from build123d import *

# Parameters (mm, degrees)
SKETCH_1_W               = 105
SKETCH_1_H               = 105
EXTRUDE_1_DEPTH          = 9
SKETCH_2_R               = 5.5
CUT_EXTRUDE_1_DEPTH      = 9
SKETCH_4_W               = 10
SKETCH_4_H               = 10
EXTRUDE_2_DEPTH          = 30
SKETCH_5_R               = 12.5
EXTRUDE_3_DEPTH          = 10
SKETCH_6_W               = 8
SKETCH_6_H               = 8
EXTRUDE_4_DEPTH          = 380
EXTRUDE_5_DEPTH          = 10
PATTERN_LINEAR_1_COUNT   = 5
PATTERN_LINEAR_1_PITCH   = 80
EXTRUDE_6_DEPTH          = 10
SKETCH_9_W               = 105
SKETCH_9_H               = 15
CUT_EXTRUDE_2_DEPTH      = 59
SPLIT_START              = -31.043560763
SPLIT_BODIES_2_OUTLINE_R = 5.5
SPLIT_BODIES_2_DEPTH     = 40.043560763
SKETCH_10_W              = 8
SKETCH_10_H              = 8
EXTRUDE_8_DEPTH          = 9


# Read off the part's stored shape, not the designer's step: 分割2
with BuildPart() as part:
    # 草图1 → 凸台-拉伸1 (new body)
    with BuildSketch(Plane(origin=(0, 0, 0), x_dir=(1, 0, 0), z_dir=(0, 1, 0))):
        with BuildLine():
            Line((-102.5, 102.5), (102.5, 102.5))
            Line((102.5, 102.5), (146.930137945, 8.550357413))
            ThreePointArc((146.930137945, 8.550357413), (148.85, 0), (146.930137945, -8.550357413))
            Line((146.930137945, -8.550357413), (90, -67.5))
            Line((90, -67.5), (52.5, -67.5))
            Line((52.5, -67.5), (-52.5, -67.5))
            Line((-52.5, -67.5), (-90, -67.5))
            Line((-90, -67.5), (-146.930137945, -8.550357413))
            ThreePointArc((-146.930137945, -8.550357413), (-148.85, 0), (-146.930137945, 8.550357413))
            Line((-146.930137945, 8.550357413), (-102.5, 102.5))
        make_face()
        Rectangle(SKETCH_1_W, SKETCH_1_H, mode=Mode.SUBTRACT)
    extrude(amount=EXTRUDE_1_DEPTH)

    # 草图2 → 切除-拉伸1 (cut)
    with BuildSketch(Plane(origin=(0, 9, 0), x_dir=(1, 0, 0), z_dir=(0, 1, 0))):
        with Locations(Location((-128.85, 0, 0), (0, 0, 270))):
            Circle(SKETCH_2_R)
        with Locations(Location((128.85, 0, 0), (0, 0, 270))):
            Circle(SKETCH_2_R)
    extrude(amount=-CUT_EXTRUDE_1_DEPTH, mode=Mode.SUBTRACT)

    # 草图4 → 凸台-拉伸2 (add)
    with BuildSketch(Plane.XZ):
        with Locations((-92, 0)):
            Rectangle(SKETCH_4_W, SKETCH_4_H)
        with Locations((92, 0)):
            Rectangle(SKETCH_4_W, SKETCH_4_H)
    extrude(amount=EXTRUDE_2_DEPTH)

    # 草图5 → 凸台-拉伸3 (add)
    with BuildSketch(Plane.ZY.offset(-87)):
        with Locations((0, -18.543560763)):
            Circle(SKETCH_5_R)
    extrude_3 = extrude(amount=-EXTRUDE_3_DEPTH)

    # 镜向1: 凸台-拉伸3 across plane
    add(extrude_3.mirror(Plane(origin=(0, 0, 0), x_dir=(0, 0, 1), z_dir=(1, 0, 0))))

    # 草图6 → 凸台-拉伸4 (add)
    with BuildSketch(Plane(origin=(0, 9, 0), x_dir=(1, 0, 0), z_dir=(0, 1, 0))):
        with Locations((-59, 0)):
            Rectangle(SKETCH_6_W, SKETCH_6_H)
        with Locations((59, 0)):
            Rectangle(SKETCH_6_W, SKETCH_6_H)
        with Locations((0, 59)):
            Rectangle(SKETCH_6_W, SKETCH_6_H)
        with Locations((0, -59)):
            Rectangle(SKETCH_6_W, SKETCH_6_H)
    extrude(amount=EXTRUDE_4_DEPTH)

    # 草图7 → 凸台-拉伸5 (add)
    with BuildSketch(Plane(origin=(0, 389, 0), x_dir=(1, 0, 0), z_dir=(0, 1, 0))):
        Polygon((-63, 4), (-63, 63), (63, 63), (63, -63), (-63, -63), align=None)
        Polygon((-55, 4), (-55, 55), (55, 55), (55, -55), (-55, -55), align=None, mode=Mode.SUBTRACT)
    extrude_5 = extrude(amount=-EXTRUDE_5_DEPTH)

    # 阵列(线性)1: 凸台-拉伸5 ×5
    with Locations(*[(0, -i * PATTERN_LINEAR_1_PITCH, 0) for i in range(1, PATTERN_LINEAR_1_COUNT)]):
        add(extrude_5)

    # 草图8 → 凸台-拉伸6 (add)
    with BuildSketch(Plane.XY.offset(4)):
        Polygon((-100, 9), (-63, 123.153405556), (-63, 149.099351502), (-108.409735963, 9), align=None)
        Polygon((108.409735963, 9), (100, 9), (63, 123.153405556), (63, 149.099351502), align=None)
    extrude(amount=-EXTRUDE_6_DEPTH)

    # 草图9 → 切除-拉伸2 (cut)
    with BuildSketch(Plane.XZ):
        with Locations((0, 60)):
            Rectangle(SKETCH_9_W, SKETCH_9_H)
    extrude(amount=-CUT_EXTRUDE_2_DEPTH, mode=Mode.SUBTRACT)

    # Split Bodies 2 outline → Split Bodies 2 (cut)
    with BuildSketch(Plane(origin=(0, 0, 0), x_dir=(1, 0, 0), z_dir=(0, 1, 0)).offset(SPLIT_START)):
        with BuildLine():
            Line((-90, -67.5), (-52.5, -67.5))
            Line((-52.5, -67.5), (-52.5, 52.5))
            Line((-52.5, 52.5), (52.5, 52.5))
            Line((52.5, 52.5), (52.5, -67.5))
            Line((52.5, -67.5), (90, -67.5))
            Line((90, -67.5), (146.930137945, -8.550357413))
            ThreePointArc((146.930137945, -8.550357413), (148.85, 0), (146.930137945, 8.550357413))
            Line((146.930137945, 8.550357413), (102.5, 102.5))
            Line((102.5, 102.5), (-102.5, 102.5))
            Line((-102.5, 102.5), (-146.930137945, 8.550357413))
            ThreePointArc((-146.930137945, 8.550357413), (-148.85, 0), (-146.930137945, -8.550357413))
            Line((-146.930137945, -8.550357413), (-90, -67.5))
        make_face()
        with Locations((-128.85, 0)):
            Circle(SPLIT_BODIES_2_OUTLINE_R, mode=Mode.SUBTRACT)
        with Locations((128.85, 0)):
            Circle(SPLIT_BODIES_2_OUTLINE_R, mode=Mode.SUBTRACT)
    extrude(amount=SPLIT_BODIES_2_DEPTH, mode=Mode.SUBTRACT)

    # 草图10 → 凸台-拉伸8 (add)
    with BuildSketch(Plane.XZ.offset(-9)):
        with Locations((-59, 0)):
            Rectangle(SKETCH_10_W, SKETCH_10_H)
        with Locations((59, 0)):
            Rectangle(SKETCH_10_W, SKETCH_10_H)
    extrude(amount=EXTRUDE_8_DEPTH)


solid = part.part
Work out the finished part from the listing and answer in its coordinate system (mm). A direction names the side the tool comes from. Give positions to 0.01 mm unless a question says otherwise; leave off trailing zeros. Order: outer loops, then holes, each group sorted by start corner. A loop starts at its lowest first (then second) coordinate and runs counter-clockwise, first axis right, second up. Notation, with made-up numbers: (0, -14.5) - (56, -14.5) arc R28 cw to (56, 13.5) - close; hole circle Ø2 at (-15.75, -10.5). An arc over 180 degrees is marked (long way). Answer as CSV lines item,"result". Start each with the question number.
Q1. The part is cut by section C-C (z = 40.5). Give the number of separate pieces and of enclosed holes in the cut face, then the cut area to 3 significant figures.
Q2. For faces 1 (the face through (-46.5, 309, -55.5)), 2 (the face through (4, 264, 59)), 3 (the face through (55.5, 299, 44.3)), 4 (the face through (-55, 210, 0)), determine the directions among +Z, -Z, +X, -X, +Y, -Y from which every point of the face is accessible in a straight line to the end or side of a thin tool.
Q3. The part is cut by section A-A (y = 247.5). Write down the section's boundary in (x, z), then the cut area to 3 significant figures.
Q4. The mould has two halves that part along Y. Classify faces 5 (the face through (-81.76, 65.28, -0.93)), 6 (the face through (-63, 305, 0)), 7 (the face through (4, 184, -59)), 8 (the face through (-46.5, 219, -55.5)): +Y half, -Y half, draft (parallel to the pull), parting line (faces both ways), or undercut.
Q5. Given pin 1 Ø1.5 at (x, y) = (-53.5, 275) entering from +Z; pin 2 Ø2.5 at (x, y) = (-60.5, 118.5) entering from -Z; pin 3 Ø9.5 at (x, z) = (102.5, -1) entering from -Y; pin 4 Ø6.5 at (y, z) = (29.5, -60) entering from +X, each flat-ended and moving along its own axis, determine where each tip first touches the part or whether it passes through.
Q6. The part is cut by section D-D (y = 33.5). Write down the section's boundary in (x, z).
Q7. Find the intervals of material crossed by L1, parallel to X at y = 139.5, z = 8.5; L2, parallel to Z at x = 70, y = 104.5, in increasing order. Write a range as [from, to].
Q8. The part is cut by section B-B (y = 109). Write down the section's boundary in (x, z).
Check result:
1,separate pieces,"10"
1,enclosed holes,"0"
1,area,"800 mm²"
2,face 1,"-Z, -X"
2,face 2,"+Z, -Z, +X"
2,face 3,"+Z, +X"
2,face 4,"+Y, -Y"
3,outline,"(-63, -4) - (-55, -4) - (-55, 4) - (-63, 4) - close; (-4, -63) - (4, -63) - (4, -55) - (-4, -55) - close; (-4, 55) - (4, 55) - (4, 63) - (-4, 63) - close; (55, -4) - (63, -4) - (63, 4) - (55, 4) - close"
3,area,"256 mm²"
4,face 5,"-Y half"
4,face 6,"draft"
4,face 7,"undercut"
4,face 8,"undercut"
5,pin 1,"passes through"
5,pin 2,"stops at z = -4"
5,pin 3,"stops at y = 9"
5,pin 4,"stops at x = 4"
6,outline,"(-100.47, -6) - (-92.06, -6) - (-92.06, 4) - (-100.47, 4) - close; (-63, -4) - (-55, -4) - (-55, 4) - (-63, 4) - close; (-4, -63) - (4, -63) - (4, -55) - (-4, -55) - close; (55, -4) - (63, -4) - (63, 4) - (55, 4) - close; (92.06, -6) - (100.47, -6) - (100.47, 4) - (92.06, 4) - close"
7,L1,"x = [-63, -55], [55, 63]"
7,L2,"z = [-6, 4]"
8,outline,"(-76, -6) - (-67.59, -6) - (-67.59, 4) - (-76, 4) - close; (-63, -4) - (-55, -4) - (-55, 4) - (-63, 4) - close; (-4, -63) - (4, -63) - (4, -55) - (-4, -55) - close; (-4, 55) - (4, 55) - (4, 63) - (-4, 63) - close; (55, -4) - (63, -4) - (63, 4) - (55, 4) - close; (67.59, -6) - (76, -6) - (76, 4) - (67.59, 4) - close"
